Geometry: see drawing. Coordinates: mm, zero at the bounding-box minimum. A direction names the side the tool comes from. Give positions to 0.01 mm unless a question says otherwise; leave off trailing zeros. Order: outer loops, then holes, each group sorted by start corner. A loop starts at its lowest first (then second) coordinate and runs counter-clockwise, first axis right, second up. Notation, with made-up numbers: M 68.5,86.5 L 127.5,86.5 A22 cw 127.5,93.5 Z; hole C 8,68.25 d6. An arc over 180 degrees is marked long. Answer as a JSON object with one key per item and string values. Group by question number.
1. Section query A-A (x = 7.5). Output: boundary loops of the cut face in (y, z).
2. Section query B-B (y = 8). Output: boundary loops of the cut face in (x, z).
3. Section query D-D (z = 7). Output: boundary loops of the cut face in (x, y), plus the area to 3 significant figures.
4. Pin query (flat end, axial travel): P1, Ø3, axis at y = 5, z = 1, coming from the +X side (3 decimals); P2, Ø6.5, axis at x = 7.5, y = 7.5, coming from the -Z side; P3, Ø4.5, axis at y = 10, z = 6.5, coming from the +X side. Return the tip coordinate at first contact, or that it passes through.
5. Material intervals for L1, parallel to Y at x = 7.5, z = 6.25; L2, parallel to X at y = 1.2, z = 4; L3, parallel to Y at x = 11.5, z = 2, sorted ascending. Write a range as [from, to].
6. Section query C-C (z = 5). Output: boundary loops of the cut face in (x, y), plus the area to 3 significant figures.
7. Set-up query: the marked faces 5, 6 and 7. Return all of +Z, -Z, +X, -X, +Y, -Y with unobstructed straight access to the full face (end or side cutting, diameter ignored); none if empty.
8. Pull-direction query (X, two-part tool) for the marked faces 1, 2, 3 and 4; classes: +X half, -X half, draft (parallel to the pull), parting line (faces both ways), or undercut.
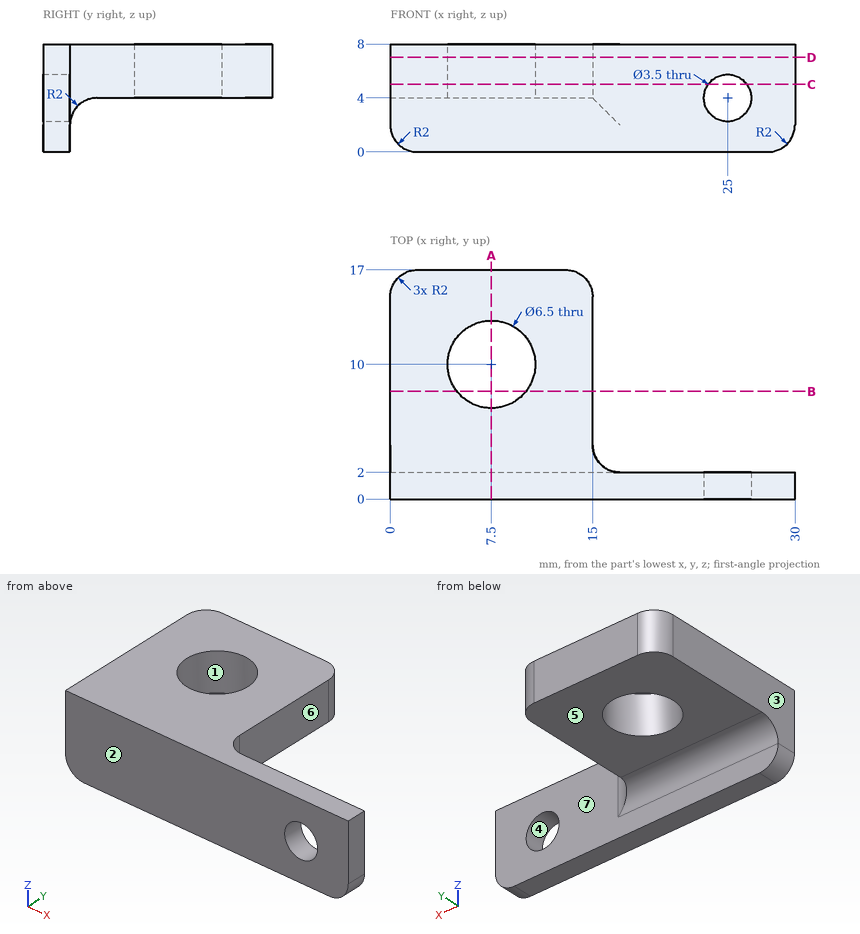
Answer sheet:
{
 "1": {"outline": "M 0,0 L 2,0 L 2,2 A2 cw 4,4 L 6.75,4 L 6.75,8 L 0,8 Z; M 13.25,4 L 17,4 L 17,8 L 13.25,8 Z"},
 "2": {"outline": "M 0,4 L 4.94,4 L 4.94,8 L 0,8 Z; M 10.06,4 L 15,4 L 15,8 L 10.06,8 Z"},
 "3": {"outline": "M 0,0 L 30,0 L 30,2 L 17,2 A2 cw 15,4 L 15,15 A2 ccw 13,17 L 2,17 A2 ccw 0,15 Z; hole C 7.5,10 d6.5", "area": "251 mm^2"},
 "4": {"P1": "through", "P2": "z = 4", "P3": "x = 15"},
 "5": {"L1": "[0, 6.75], [13.25, 17]", "L2": "[0, 23.25], [26.75, 30]", "L3": "[0, 2]"},
 "6": {"outline": "M 0,0 L 23.56,0 L 23.56,2 L 17,2 A2 cw 15,4 L 15,15 A2 ccw 13,17 L 2,17 A2 ccw 0,15 Z; M 26.44,0 L 30,0 L 30,2 L 26.44,2 Z; hole C 7.5,10 d6.5", "area": "245 mm^2"},
 "7": {"face 5": "-Z, +X, -X, +Y", "face 6": "+Z, -Z, +X, +Y", "face 7": "-Z, +X, +Y"},
 "8": {"face 1": "undercut", "face 2": "draft", "face 3": "-X half", "face 4": "undercut"}
}
